Autodesk Inventor part; units mm, degrees
ref_plane "YZ Plane" through (0, 0, 0) normal (1, 0, 0) x (0, 1, 0)
ref_plane "XZ Plane" through (0, 0, 0) normal (0, 1, 0) x (-1, 0, 0)
ref_plane "XY Plane" through (0, 0, 0) normal (0, 0, 1) x (1, 0, 0)
sketch "Sketch1" plane through (0, 0, 0) normal (0, 0, 1) x (1, 0, 0)
  circle A0 centre (0.002, 0.003) radius 2
  line L0 (-11.748, 11.753) -> (11.752, 11.753)
  line L1 (11.752, 11.753) -> (11.752, -11.747)
  line L2 (11.752, -11.747) -> (-11.748, -11.747)
  line L3 (-11.748, -11.747) -> (-11.748, 11.753)
  dimension "d5" = 4
  dimension "d8" = 23.5
  dimension "d9" = 23.5
extrude "Extrusion1" add sketch "Sketch1" along normal blind 3
properties part number "bold holder" material "Silver"
Can you work these out from the model? Positions are in its coordinate system, mm. Give positions to 0.01 mm unless a question says otherwise; leave off trailing zeros. Loops run counter-clockwise (first coordinate to the right, second up) from the corner with the lowest first, then second, coordinate; pieces in that order, holes last. Notation, with made-up numbers: (24.5, 57.5) -> (67.5, 57.5) arc R10 cw to (67.5, 69.5) -> close; hole circle Ø8 at (62, 60). An arc over 180 degrees is marked (long way). Use one line per item in the form item = value.
1) I need wall thicknesses on line 1 along X through (y, z) = (-0.5, 0.45); line 2 along Y through (x, z) = (0.75, 2.45); line 3 along X through (y, z) = (-1.25, 1.9). Which ranges of each line are inside material? Lowest first, please.
Answers:
line_1 = -11.75 to -1.93, 1.94 to 11.75
line_2 = -11.75 to -1.85, 1.86 to 11.75
line_3 = -11.75 to -1.56, 1.56 to 11.75
2) Will these pins go through, and if not, where does the flat tip stop? pin 1 (2.5 mm diameter, centred on x = 0.002, y = 0.003, fed in from -Z); pin 2 (1.5 mm diameter, centred on x = -6.5, y = 8.5, fed in from -Z).
Answers:
pin_1 = through
pin_2 = 0
3) If we section it at C-C (z = 2.5): Please give me the cut outline in (x, y).
Answers:
outline = (-11.75, -11.75) -> (11.75, -11.75) -> (11.75, 11.75) -> (-11.75, 11.75) -> close; hole circle Ø4 at (0, 0)
4) We'd pull the mould along X, two halves only. Please class faces 1 (the face through (-0.432, 1.955, 1.479)), 2 (the face through (11.752, 0, 1)), 3 (the face through (2.4, 0.2, 3)), 4 (the face through (-11.748, 0, 1)): released by +X, released by -X, zero draft, split by the parting line, or undercut.
Answers:
face_1 = undercut
face_2 = released by +X
face_3 = zero draft
face_4 = released by -X
5) If we section it at A-A (y = -1.5): Please give me the cut outline in (x, z), plus the area to 3 significant figures.
Answers:
outline = (-11.75, 0) -> (-1.32, 0) -> (-1.32, 3) -> (-11.75, 3) -> close; (1.32, 0) -> (11.75, 0) -> (11.75, 3) -> (1.32, 3) -> close
area = 62.6 mm²
